The listing builds one solid part. Answer for the finished solid, in the listing's coordinates (mm). Face numbers are marked on the shaded views. A direction names the side the tool comes from. Round coordinates to 2 decimals unless told otherwise and drop trailing zeros. Loops run counter-clockwise (first coordinate to the right, second up) from the corner with the lowest first, then second, coordinate; pieces in that order, holes last. Notation, with made-up numbers: M -27.75,-10 L -7.75,-10 A15 ccw -7.75,-3 Z; hole C 32,74.5 d10. An arc over 180 degrees is marked long. Put each result on its own line as item: value. Start each with the question number.
(1) Section A-A, the plane z = -3 is taken. Determine the outline of the cut face in (x, y), then the cut area to 3 significant figures.
(2) Flat-ended cylindrical pins translate along their axes: P1, Ø1.5, axis at x = 15, y = 18, coming from the -Z side; P2, Ø0.6, axis at x = 19.5, y = 22.5, coming from the +Z side. Find the tip coordinate at first contact, or state that the pin passes through.
(3) Straight lines are drawn through the part: line 1 (X direction, y = 13, z = -1.75); line 2 (X direction, y = 2, z = -14.5); line 3 (Z direction, x = 5.5, y = 16). For each, find the intervals that lie inside material, in ascending order.
(4) Determine the mould class of the marked faces 3, 4, 5 and 6 for opening direction X: released by +X, released by -X, zero draft, split by the parting line, or undercut.
(5) Section C-C, the plane y = 24.5 is taken. Determine the outline of the cut face in (x, z), then the cut area to 3 significant figures.
(6) Section B-B, the plane z = -12.25 is taken. Determine the outline of the cut face in (x, y), then the cut area to 3 significant figures.
(7) Which of the six approach directions +Z, -Z, +X, -X, +Y, -Y give full straight-line access (tool end or side, diameter ignored) to the marked faces 1 and 2?
```python
from build123d import *

# Parameters (mm, degrees)
BOSS_EXTRUDE1_DEPTH = 31
SKETCH2_W           = 2
SKETCH2_H           = 4.533544861
CUT_EXTRUDE1_DEPTH  = 32


with BuildPart() as part:
    # Sketch1 → Boss-Extrude1 (new body)
    with BuildSketch(Plane(origin=(0, 0, 0), x_dir=(1, 0, 0), z_dir=(0, 1, 0))):
        Polygon((21.4, 16), (23.4, 16), (23.4, 0), (0, 0), (0, 16), (2, 16), (2, 9), (21.4, 9), align=None)
    extrude(amount=BOSS_EXTRUDE1_DEPTH)

    # Sketch2 → Cut-Extrude1 (cut, through all)
    with BuildSketch(Plane(origin=(0, 31, 0), x_dir=(1, 0, 0), z_dir=(0, 1, 0))):
        with Locations((3.766668881, 2.266772431)):
            Rectangle(SKETCH2_W, SKETCH2_H)
        with Locations((7.766668881, 2.266772431)):
            Rectangle(SKETCH2_W, SKETCH2_H)
        with Locations((11.766668881, 2.266772431)):
            Rectangle(SKETCH2_W, SKETCH2_H)
        with Locations((15.766668881, 2.266772431)):
            Rectangle(SKETCH2_W, SKETCH2_H)
        with Locations((19.766668881, 2.266772431)):
            Rectangle(SKETCH2_W, SKETCH2_H)
    extrude(amount=-CUT_EXTRUDE1_DEPTH, mode=Mode.SUBTRACT)


solid = part.part
```
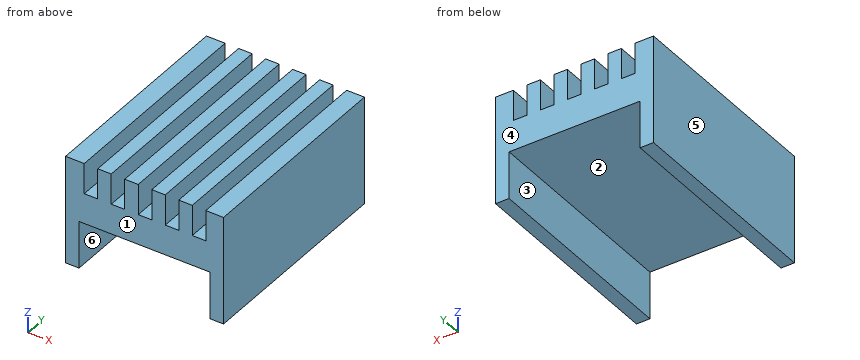
Recorded:
1. outline: M 0,0 L 2.77,0 L 2.77,31 L 0,31 Z; M 4.77,0 L 6.77,0 L 6.77,31 L 4.77,31 Z; M 8.77,0 L 10.77,0 L 10.77,31 L 8.77,31 Z; M 12.77,0 L 14.77,0 L 14.77,31 L 12.77,31 Z; M 16.77,0 L 18.77,0 L 18.77,31 L 16.77,31 Z; M 20.77,0 L 23.4,0 L 23.4,31 L 20.77,31 Z
1. area: 415 mm²
2. P1: stops at z = -9
2. P2: stops at z = -4.53
3. line 1: x = 0 to 2.77, 4.77 to 6.77, 8.77 to 10.77, 12.77 to 14.77, 16.77 to 18.77, 20.77 to 23.4
3. line 2: x = 0 to 2, 21.4 to 23.4
3. line 3: z = -9 to 0
4. face 3: undercut
4. face 4: zero draft
4. face 5: released by -X
4. face 6: undercut
5. outline: M 0,-16 L 2,-16 L 2,-9 L 21.4,-9 L 21.4,-16 L 23.4,-16 L 23.4,0 L 20.77,0 L 20.77,-4.53 L 18.77,-4.53 L 18.77,0 L 16.77,0 L 16.77,-4.53 L 14.77,-4.53 L 14.77,0 L 12.77,0 L 12.77,-4.53 L 10.77,-4.53 L 10.77,0 L 8.77,0 L 8.77,-4.53 L 6.77,-4.53 L 6.77,0 L 4.77,0 L 4.77,-4.53 L 2.77,-4.53 L 2.77,0 L 0,0 Z
5. area: 193 mm²
6. outline: M 0,0 L 2,0 L 2,31 L 0,31 Z; M 21.4,0 L 23.4,0 L 23.4,31 L 21.4,31 Z
6. area: 124 mm²
7. face 1: +Z, -Z, +X, -X, -Y
7. face 2: -Z, +Y, -Y
